from build123d import *

# Parameters (mm, degrees)
SCHIZZO1_R                   = 2.5
SCHIZZO1_R_2                 = 1.75
ESTRUSIONE_ESTRUSIONE1_DEPTH = 3


with BuildPart() as part:
    # Schizzo1 → Estrusione-Estrusione1 (new body)
    with BuildSketch(Plane.XY):
        with BuildLine():
            Line((0, 0), (0, 449))
            Line((0, 449), (164.5, 449))
            Line((164.5, 449), (164.5, 419))
            ThreePointArc((164.5, 419), (167.428932188, 411.928932188), (174.5, 409))
            Line((174.5, 409), (274.5, 409))
            ThreePointArc((274.5, 409), (281.571067812, 411.928932188), (284.5, 419))
            Line((284.5, 419), (284.5, 449))
            Line((284.5, 449), (449, 449))
            Line((449, 449), (449, 0))
            Line((449, 0), (0, 0))
        make_face()
        with Locations((11.5, 11.5)):
            Circle(SCHIZZO1_R, mode=Mode.SUBTRACT)
        with Locations(Location((437.5, 11.5, 0), (0, 0, 180))):
            Circle(SCHIZZO1_R, mode=Mode.SUBTRACT)
        with Locations((437.5, 437.5)):
            Circle(SCHIZZO1_R, mode=Mode.SUBTRACT)
        with Locations(Location((11.5, 437.5, 0), (0, 0, 180))):
            Circle(SCHIZZO1_R, mode=Mode.SUBTRACT)
        with Locations((319.5, 399)):
            Circle(SCHIZZO1_R_2, mode=Mode.SUBTRACT)
        with BuildLine():
            Line((344.715899345, 409), (405.440355678, 409))
            ThreePointArc((405.440355678, 409), (415.440355678, 399), (405.440355678, 389))
            Line((405.440355678, 389), (344.715899345, 389))
            ThreePointArc((344.715899345, 389), (334.715899345, 399), (344.715899345, 409))
        make_face(mode=Mode.SUBTRACT)
    extrude(amount=ESTRUSIONE_ESTRUSIONE1_DEPTH)


solid = part.part
The listing builds one solid part. Answer for the finished solid, in the listing's coordinates (mm). A direction names the side the tool comes from. Give positions to 0.01 mm unless a question says otherwise; leave off trailing zeros. Order: outer loops, then holes, each group sorted by start corner. A loop starts at its lowest first (then second) coordinate and runs counter-clockwise, first axis right, second up. Notation, with made-up numbers: (10.5, 57) - (24.5, 57) arc R16 cw to (24.5, 79) - close; hole circle Ø2 at (47, 67). An arc over 180 degrees is marked (long way). One line per item, written item: value. Start each with the question number.
1) A cutting plane is placed at B-B on z = 2.3. Give the vertices of the cut face in (x, y), then the cut area to 3 significant figures.
2) Find the intervals of material crossed by L1, parallel to Y at x = 11.5, z = 1.3; L2, parallel to X at y = 399, z = 0.75; L3, parallel to X at y = 423, z = 1.5, in increasing order.
3) A tool of negligible diameter and unlimited length cuts with its end or side. For faces 3 (the face through (228, 228, 0)), 4 (the face through (334.72, 398.78, 1.48)), 5 (the face through (281.49, 411.85, 1.48)), from which of +Z, -Z, +X, -X, +Y, -Y can it reach the whole face along a straight path? Write none if from no direction.
4) A cutting plane is placed at C-C on x = 201. Give the vertices of the cut face in (y, z).
5) Given pin 1 Ø6.5 at (x, y) = (11.5, 437.5) entering from -Z; pin 2 Ø4.5 at (x, y) = (11.5, 11.5) entering from -Z; pin 3 Ø0.9 at (x, z) = (222.5, 1) entering from +Y, each flat-ended and moving along its own axis, determine where each tip first touches the part or whether it passes through.
6) A cutting plane is placed at A-A on x = 400. Give the vertices of the cut face in (y, z).
7) The mould has two halves that part along X. Classify faces 1 (the face through (167.35, 412.01, 1.48)), 2 (the face through (228, 228, 3)): released by +X, released by -X, zero draft, split by the parting line, or undercut.
Answer sheet:
1. outline: (0, 0) - (449, 0) - (449, 449) - (284.5, 449) - (284.5, 419) arc R10 cw to (274.5, 409) - (174.5, 409) arc R10 cw to (164.5, 419) - (164.5, 449) - (0, 449) - close; hole circle Ø5 at (11.5, 11.5); hole circle Ø5 at (11.5, 437.5); hole circle Ø3.5 at (319.5, 399); hole (344.72, 389) - (405.44, 389) arc R10 ccw to (405.44, 409) - (344.72, 409) arc R10 ccw to start; hole circle Ø5 at (437.5, 11.5); hole circle Ø5 at (437.5, 437.5)
1. area: 195,000 mm2
2. L1: y = 0 to 9, 14 to 435, 440 to 449
2. L2: x = 0 to 317.75, 321.25 to 334.72, 415.44 to 449
2. L3: x = 0 to 164.5, 284.5 to 449
3. face 3: -Z, +X, -X, +Y, -Y
3. face 4: +Z, -Z
3. face 5: +Z, -Z, +Y
4. outline: (0, 0) - (409, 0) - (409, 3) - (0, 3) - close
5. pin 1: stops at z = 0
5. pin 2: passes through
5. pin 3: stops at y = 409
6. outline: (0, 0) - (389, 0) - (389, 3) - (0, 3) - close; (409, 0) - (449, 0) - (449, 3) - (409, 3) - close
7. face 1: undercut
7. face 2: zero draft
